The model under review builds one solid part; all positions refer to its coordinate system, in mm. Face numbers are marked on the shaded views. A direction names the side the tool comes from. Round coordinates to 2 decimals unless told otherwise and drop trailing zeros. Loops run counter-clockwise (first coordinate to the right, second up) from the corner with the lowest first, then second, coordinate; pieces in that order, holes last. Notation, with made-up numbers: (1, -24.75) -> (21, -24.75) arc R20 ccw to (21, -13.75) -> close; hole circle Ø9 at (82, 54). An arc over 180 degrees is marked (long way). Return JSON: item names as keys, results as strings. Group by question number.
```python
from build123d import *

# Parameters (mm, degrees)
CROQUIS1_W              = 50.8
CROQUIS1_H              = 76.2
SALIENTE_EXTRUIR1_DEPTH = 18
CROQUIS2_W              = 50.8
CROQUIS2_H              = 76.2
CROQUIS2_W_2            = 46.12
CROQUIS2_H_2            = 71.52
CROQUIS2_W_3            = 38.8
CROQUIS2_H_3            = 64.2
CORTAR_EXTRUIR1_DEPTH   = 15
CORTAR_EXTRUIR8_DEPTH   = 15
SALIENTE_EXTRUIR3_DEPTH = 41.5
CORTAR_EXTRUIR9_DEPTH   = 51.5
CORTAR_EXTRUIR10_DEPTH  = 51.5
SALIENTE_EXTRUIR4_DEPTH = 16
CORTAR_EXTRUIR11_DEPTH  = 16.5
REDONDEO3_R             = 2
REDONDEO4_R             = 1
CROQUIS15_W             = 48.12
CROQUIS15_H             = 10
CORTAR_EXTRUIR12_DEPTH  = 15
CROQUIS16_W             = 8
CROQUIS16_H             = 1.5
CORTAR_EXTRUIR13_DEPTH  = 2
CROQUIS18_R             = 1.5
CROQUIS18_W             = 17
CROQUIS18_H             = 10
CROQUIS18_W_2           = 15
CORTAR_EXTRUIR15_DEPTH  = 3
CORTAR_EXTRUIR16_DEPTH  = 10


with BuildPart() as part:
    # Croquis1 → Saliente-Extruir1 (new body)
    with BuildSketch(Plane.XY):
        Rectangle(CROQUIS1_W, CROQUIS1_H)
    extrude(amount=SALIENTE_EXTRUIR1_DEPTH)

    # Croquis2 → Cortar-Extruir1 (cut)
    # profile 1 of 2: a face of its own
    with BuildSketch(Plane.XY.offset(18)):
        Rectangle(CROQUIS2_W, CROQUIS2_H)
        Rectangle(CROQUIS2_W_2, CROQUIS2_H_2, mode=Mode.SUBTRACT)
    # profile 2 of 2: a face of its own
    with BuildSketch(Plane.XY.offset(18)):
        Rectangle(CROQUIS2_W_3, CROQUIS2_H_3)
    extrude(amount=-CORTAR_EXTRUIR1_DEPTH, mode=Mode.SUBTRACT)

    # Croquis6 → Cortar-Extruir8 (cut)
    with BuildSketch(Plane.XY.offset(18)):
        Polygon((-23.06, 35.76), (-8.06, 35.76), (-8.06, 32.1), (-19.4, 32.1), (-19.4, 20.76), (-23.06, 20.76), align=None)
        Polygon((23.06, 35.76), (8.06, 35.76), (8.06, 32.1), (19.4, 32.1), (19.4, 20.76), (23.06, 20.76), align=None)
        Polygon((-23.06, -35.76), (-23.06, -20.76), (-19.4, -20.76), (-19.4, -32.1), (-8.06, -32.1), (-8.06, -35.76), align=None)
        Polygon((23.06, -35.76), (8.06, -35.76), (8.06, -32.1), (19.4, -32.1), (19.4, -20.76), (23.06, -20.76), align=None)
    extrude(amount=-CORTAR_EXTRUIR8_DEPTH, mode=Mode.SUBTRACT)

    # Croquis10 → Saliente-Extruir3 (add)
    with BuildSketch(Plane(origin=(0, -20.76, 0), x_dir=(-1, 0, 0), z_dir=(0, -1, 0))):
        Polygon((23.06, -18), (24.06, -18), (23.06, -3), align=None)
        Polygon((-23.06, -18), (-24.06, -18), (-23.06, -3), align=None)
    extrude(amount=-SALIENTE_EXTRUIR3_DEPTH)

    # Croquis11 → Cortar-Extruir9 (cut)
    with BuildSketch(Plane.XZ.offset(20.76)):
        Polygon((-19.4, 18), (-21.56, 18), (-20.56, 3), (-19.4, 3), align=None)
    extrude(amount=-CORTAR_EXTRUIR9_DEPTH, mode=Mode.SUBTRACT)

    # Croquis12 → Cortar-Extruir10 (cut)
    with BuildSketch(Plane.XZ.offset(20.76)):
        Polygon((19.4, 18), (19.4, 3), (20.56, 3), (21.56, 18), align=None)
    extrude(amount=-CORTAR_EXTRUIR10_DEPTH, mode=Mode.SUBTRACT)

    # Croquis13 → Saliente-Extruir4 (add)
    with BuildSketch(Plane(origin=(8.06, 0, 0), x_dir=(0, 0, -1), z_dir=(1, 0, 0))):
        Polygon((-18, -35.76), (-18, -37.76), (-3, -35.76), align=None)
        Polygon((-18, 35.76), (-18, 37.76), (-3, 35.76), align=None)
    extrude(amount=-SALIENTE_EXTRUIR4_DEPTH)

    # Croquis14 → Cortar-Extruir11 (cut)
    with BuildSketch(Plane(origin=(8.06, 0, 0), x_dir=(0, 0, -1), z_dir=(1, 0, 0))):
        Polygon((-3, -32.1), (-18, -32.1), (-18, -35.26), (-3, -33.26), align=None)
        Polygon((-18, 32.1), (-18, 35.26), (-3, 33.26), (-3, 32.1), align=None)
    extrude(amount=-CORTAR_EXTRUIR11_DEPTH, mode=Mode.SUBTRACT)

    # Redondeo3
    redondeo3_edges = [part.edges().sort_by_distance(p)[0] for p in [
        (-25.4, 38.1, 1.5),
        (25.4, 38.1, 1.5),
        (25.4, -38.1, 1.5),
        (-25.4, -38.1, 1.5),
    ]]
    fillet(redondeo3_edges, radius=REDONDEO3_R)

    # Redondeo4
    redondeo4_edges = [part.edges().sort_by_distance(p)[0] for p in [
        (0, 38.1, 0),
        (-25.4, 0, 0),
        (25.4, 0, 0),
        (0, -38.1, 0),
        (24.814213562, -37.514213562, 0),
        (-24.814213562, -37.514213562, 0),
        (-24.814213562, 37.514213562, 0),
        (24.814213562, 37.514213562, 0),
    ]]
    fillet(redondeo4_edges, radius=REDONDEO4_R)

    # Croquis15 → Cortar-Extruir12 (cut)
    with BuildSketch(Plane.XY.offset(18)):
        with Locations((0, -0.01)):
            Rectangle(CROQUIS15_W, CROQUIS15_H)
    extrude(amount=-CORTAR_EXTRUIR12_DEPTH, mode=Mode.SUBTRACT)

    # Croquis16 → Cortar-Extruir13 (cut)
    with BuildSketch(Plane.XZ.offset(38.1)):
        with Locations((0, 2.25)):
            Rectangle(CROQUIS16_W, CROQUIS16_H)
    extrude(amount=-CORTAR_EXTRUIR13_DEPTH, mode=Mode.SUBTRACT)

    # Croquis18 → Cortar-Extruir15 (cut)
    with BuildSketch(Plane.XY.offset(3)):
        with Locations((1.1, 0)):
            Circle(CROQUIS18_R)
        with Locations((1.1, 25)):
            Circle(CROQUIS18_R)
        with Locations((1.1, -25)):
            Circle(CROQUIS18_R)
        with Locations((-9.9, 0.1)):
            Rectangle(CROQUIS18_W, CROQUIS18_H)
        with Locations((11.1, 0.1)):
            Rectangle(CROQUIS18_W_2, CROQUIS18_H)
    extrude(amount=-CORTAR_EXTRUIR15_DEPTH, mode=Mode.SUBTRACT)

    # Croquis19 → Cortar-Extruir16 (cut)
    with BuildSketch(Plane.XY.offset(3)):
        with BuildLine():
            Line((25.4, -32.419906808), (17.4, -32.419906808))
            ThreePointArc((17.4, -32.419906808), (14.9, -29.919906808), (17.4, -27.419906808))
            Line((17.4, -27.419906808), (25.4, -27.419906808))
            ThreePointArc((25.4, -27.419906808), (27.9, -29.919906808), (25.4, -32.419906808))
        make_face()
    extrude(amount=-CORTAR_EXTRUIR16_DEPTH, mode=Mode.SUBTRACT)


solid = part.part
```
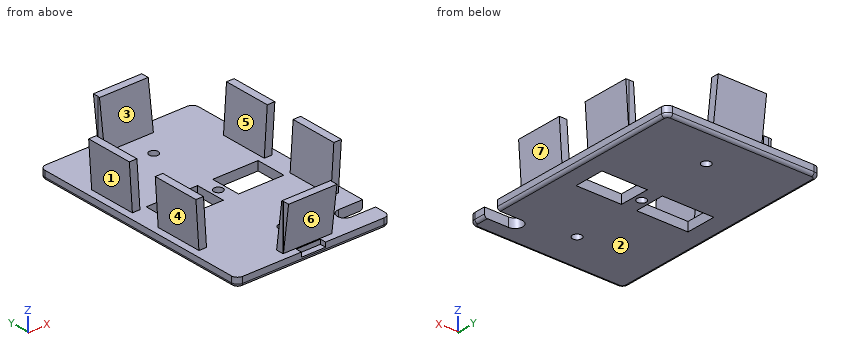
1. Wall thickness on line 1 (Y direction, x = 1.1, z = 1); line 2 (Y direction, x = 1.1, z = 1.8); line 3 (Y direction, x = -22, z = 3.5): over which ranges is each line inside the solid? List them lowest first.
2. We need section B-B, the plane z = 9. Give the number of separate pieces and of enclosed holes in the cut face, then the cut area to 3 significant figures.
3. We need section D-D, the plane y = -25. Write out the cut boundary in (x, z).
4. We need section C-C, the plane y = 3. Write out the cut boundary in (x, z).
5. Tool access review of the marked faces 5, 6 and 7: name each direction out of +Z, -Z, +X, -X, +Y, -Y from which nothing blocks a thin tool from reaching the whole face with its end or side.
6. Draft analysis for pull direction Z (two halves, no side actions). For the marked faces 1, 2, 3 and 4, state which applies: pulls with the +Z half, pulls with the -Z half, needs draft (parallel to the pull), parting line crosses it, or undercut.
7. We need section A-A, the plane x = -3. Write out the cut boundary in (y, z), then the cut area to 3 significant figures.
8. For P1, Ø15, axis at x = 3.5, y = 17.5, coming from the +Z side; P2, Ø2, axis at y = 34, z = 13, coming from the -X side; P3, Ø3, axis at x = -20, z = 10, coming from the +Y side, all flat-tipped, find the tip position at first contact; note any pin that passes through.
Check sheet entries:
{
 "1": {"line 1": "y = -38.1 to -26.5, -23.5 to -1.5, 1.5 to 23.5, 26.5 to 38.1", "line 2": "y = -36.1 to -26.5, -23.5 to -1.5, 1.5 to 23.5, 26.5 to 38.1", "line 3": "y = -20.76 to -5.01, 4.99 to 20.76"},
 "2": {"separate pieces": "6", "enclosed holes": "0", "area": "238 mm²"},
 "3": {"outline": "(-25.4, 1) arc R1 ccw to (-24.4, 0) -> (-0.4, 0) -> (-0.4, 3) -> (-25.4, 3) -> close; (2.6, 0) -> (24.4, 0) arc R1 ccw to (25.4, 1) -> (25.4, 3) -> (2.6, 3) -> close"},
 "4": {"outline": "(-25.4, 1) arc R1 ccw to (-24.4, 0) -> (-18.4, 0) -> (-18.4, 3) -> (-25.4, 3) -> close; (-1.4, 0) -> (3.6, 0) -> (3.6, 3) -> (-1.4, 3) -> close; (18.6, 0) -> (24.4, 0) arc R1 ccw to (25.4, 1) -> (25.4, 3) -> (18.6, 3) -> close"},
 "5": {"face 5": "+Z, +Y, -Y", "face 6": "+X, -X, -Y", "face 7": "+X, +Y, -Y"},
 "6": {"face 1": "undercut", "face 2": "pulls with the -Z half", "face 3": "pulls with the +Z half", "face 4": "undercut"},
 "7": {"outline": "(-38.1, 1) arc R1 ccw to (-37.1, 0) -> (-4.9, 0) -> (-4.9, 3) -> (-33.26, 3) -> (-35.26, 18) -> (-37.76, 18) -> (-35.76, 3) -> (-36.1, 3) -> (-36.1, 1.5) -> (-38.1, 1.5) -> close; (5.1, 0) -> (37.1, 0) arc R1 ccw to (38.1, 1) -> (38.1, 3) -> (35.76, 3) -> (37.76, 18) -> (35.26, 18) -> (33.26, 3) -> (5.1, 3) -> close", "area": "270 mm²"},
 "8": {"P1": "stops at z = 3", "P2": "stops at x = -8.06", "P3": "stops at y = 20.76"}
}
